Could you check a few things on this model? Use its own coordinates, in mm. Face numbers are marked on the shaded views. A direction names the side the tool comes from. Round coordinates to 2 decimals unless told otherwise and drop trailing zeros. Loops run counter-clockwise (first coordinate to the right, second up) from the corner with the lowest first, then second, coordinate; pieces in that order, holes last. Notation, with made-up numbers: (56.5, -26) - (77.5, -26) arc R17 ccw to (77.5, -6) - close; hole circle Ø8 at (57, 61). An arc over 180 degrees is marked (long way). Use one line per item in the form item = value.
```python
from build123d import *

# Parameters (mm, degrees)
BOSS_EXTRUDE1_DEPTH = 111.092
SKETCH3_R           = 12.7
BOSS_EXTRUDE2_DEPTH = 25.4
SKETCH4_R           = 31.75
SKETCH4_R_2         = 19.05
BOSS_EXTRUDE3_DEPTH = 86.106


with BuildPart() as part:
    # Sketch2 → Boss-Extrude1 (new body)
    with BuildSketch(Plane(origin=(0, 0, 0), x_dir=(1, 0, 0), z_dir=(0, 1, 0))):
        Polygon((101.6, 0), (0, 0), (0, -177.8), (12.7, -177.8), (12.7, -12.7), (101.6, -12.7), align=None)
    extrude(amount=BOSS_EXTRUDE1_DEPTH)

    # Sketch3 → Boss-Extrude2 (add)
    with BuildSketch(Plane(origin=(0, 0, 0), x_dir=(-1, 0, 0), z_dir=(0, 0, -1))):
        with Locations((-50.8, 55.546)):
            Circle(SKETCH3_R)
    extrude(amount=BOSS_EXTRUDE2_DEPTH)

    # Sketch4 → Boss-Extrude3 (add)
    with BuildSketch(Plane(origin=(12.7, 0, 0), x_dir=(0, 0, -1), z_dir=(1, 0, 0))):
        with Locations(Location((-127, 55.546, 0), (0, 0, 180))):
            Circle(SKETCH4_R)
        with Locations((-127, 55.546)):
            Circle(SKETCH4_R_2, mode=Mode.SUBTRACT)
    extrude(amount=BOSS_EXTRUDE3_DEPTH)


solid = part.part
```
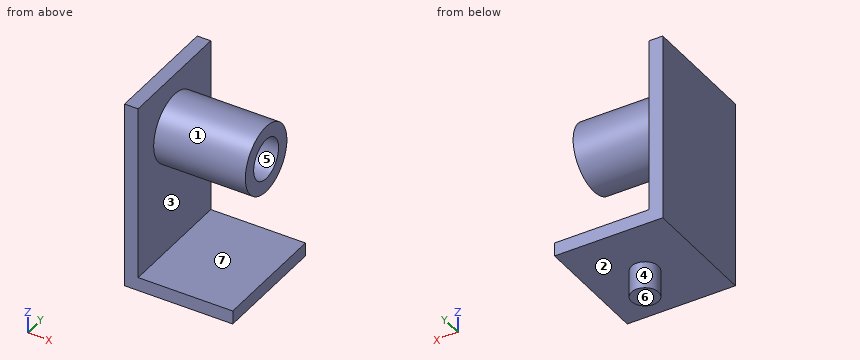
1. If we section it at C-C, the plane y = 10: Write out the boundary of the cut face in (x, z), plus the area to 3 significant figures.
Solution:
outline = (0, 0) - (101.6, 0) - (101.6, 12.7) - (12.7, 12.7) - (12.7, 177.8) - (0, 177.8) - close
area = 3,390 mm^2
2. We'd pull the mould along Z, two halves only. Please class the marked faces 1, 2, 3 and 4: +Z half, -Z half, draft (parallel to the pull), parting line (faces both ways), or undercut.
Solution:
face_1 = undercut
face_2 = -Z half
face_3 = undercut
face_4 = draft
3. If we section it at B-B, the plane z = 127: Write out the boundary of the cut face in (x, y).
Solution:
outline = (0, 0) - (12.7, 0) - (12.7, 23.8) - (98.81, 23.8) - (98.81, 36.5) - (12.7, 36.5) - (12.7, 74.6) - (98.81, 74.6) - (98.81, 87.3) - (12.7, 87.3) - (12.7, 111.09) - (0, 111.09) - close
4. If we section it at A-A, the plane x = 44.5: Write out the boundary of the cut face in (y, z), plus the area to 3 significant figures.
Solution:
outline = (0, 0) - (44.52, 0) - (44.52, -25.4) - (66.57, -25.4) - (66.57, 0) - (111.09, 0) - (111.09, 12.7) - (0, 12.7) - close; circle Ø63.5 at (55.55, 127); hole circle Ø38.1 at (55.55, 127)
area = 4,000 mm^2
5. Please list where these lines run through material, in increasing order: line 1 along Z through (x, y) = (26.5, 54.5); line 2 along Y through (x, z) = (75, 127); line 3 along X through (y, z) = (94.5, 160.5).
Solution:
line_1 = 0 to 12.7, 95.27 to 107.98, 146.02 to 158.73
line_2 = 23.8 to 36.5, 74.6 to 87.3
line_3 = 0 to 12.7
6. On a 3-axis mill with a long thin cutter (end or side, diameter ignored), from which of +Z, -Z, +X, -X, +Y, -Y can I reach the whole of each face in a straight line? I mean the marked faces 5, 6 and 7. Say none if no direction works.
Solution:
face_5 = +X
face_6 = -Z, +X, -X, +Y, -Y
face_7 = +X, +Y, -Y
7. For P1, Ø8, axis at x = 23.5, z = -2, coming from the +Y side; P2, Ø10, axis at x = 27, y = 53, coming from the -Z side; P3, Ø8, axis at x = 69, y = 87, coming from the +Z side; P4, Ø1, axis at x = 30.5, y = 77.5, coming from the +Z side, each with a flat end and sliding along its axis, tell me the tip position at first contact or that it passes through.
Solution:
P1 = 111.09
P2 = 0
P3 = 142.95
P4 = 150.4
8. If we section it at D-D, the plane x = 76.5: Write out the boundary of the cut face in (y, z).
Solution:
outline = (0, 0) - (111.09, 0) - (111.09, 12.7) - (0, 12.7) - close; circle Ø63.5 at (55.55, 127); hole circle Ø38.1 at (55.55, 127)
